Answer from the drawing. Dimensions are ordinates in mm from the lowest x, y and z of the part. A direction names the side the tool comes from. Give positions to 0.01 mm unless a question says otherwise; leave off trailing zeros. Write each loop counter-clockwise with the first axis right and the second up, starting at its lowest first coordinate (ties: lowest second). Pieces come first, ordered by that corner, then holes. Notation, with made-up numbers: (26, 84) -> (49, 84) arc R20 ccw to (49, 88) -> close; hole circle Ø1 at (-20.5, -10). An arc over 180 degrees is marked (long way). Write item = value, one per line.
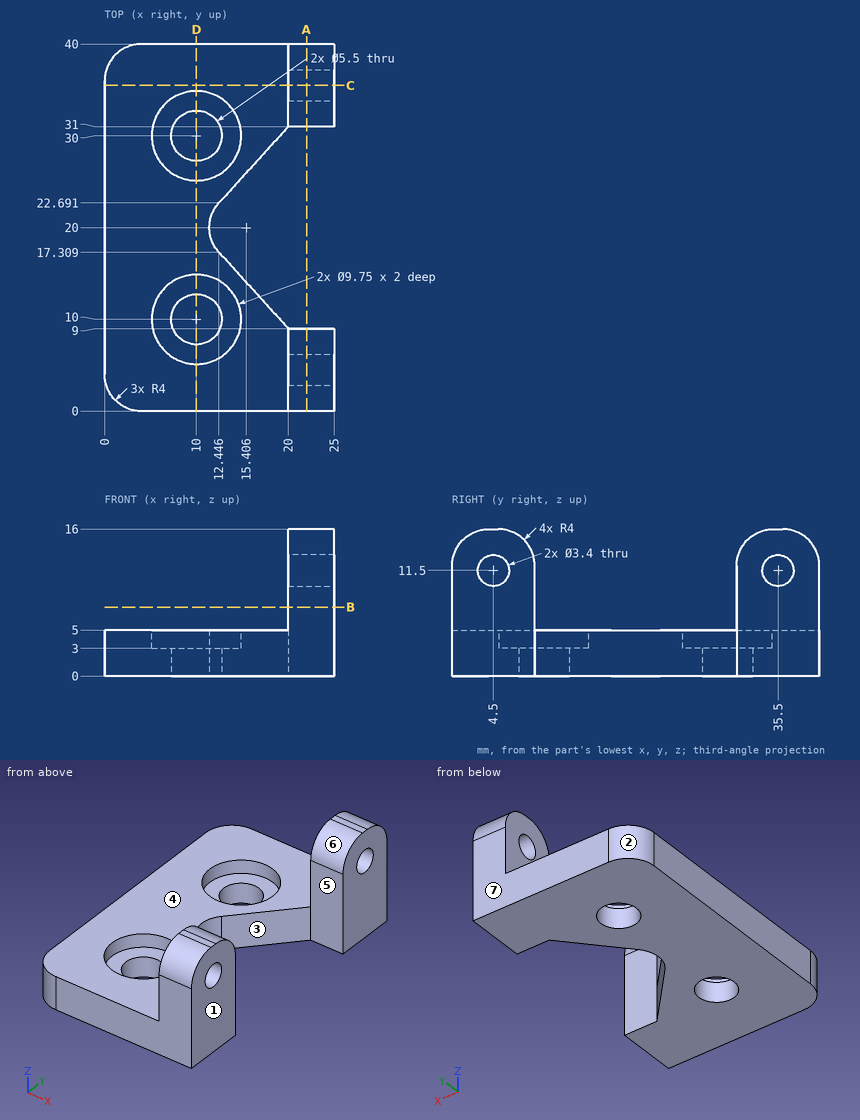
(1) The part is cut by section D-D on x = 10. Count the separate pieces of the cut face and the enclosed holes in it, plus the area to 3 significant figures.
Checks:
separate_pieces = 3
enclosed_holes = 0
area = 128 mm²
(2) A tool of negligible diameter and unlimited length cuts with its end or side. For the marked faces 4, 5, 6 and 7, from which of +Z, -Z, +X, -X, +Y, -Y can it reach the whole face along a straight path? Write none if from no direction.
Checks:
face_4 = +Z, -X, +Y, -Y
face_5 = +Z, -Z, +X
face_6 = +Z, +X, -X
face_7 = +Z, -Z, +X, -X, +Y
(3) Consider L1, parallel to Y at x = 23.7, z = 11.5; L2, parallel to Y at x = 22, z = 1; L3, parallel to Y at x = 12, z = 1.5 (1 decimal). Determine where each line is inside the solid, lowest interval first.
Checks:
L1 = 0 to 2.8, 6.2 to 9, 31 to 33.8, 37.2 to 40
L2 = 0 to 9, 31 to 40
L3 = 0 to 8.1, 11.9 to 17.9, 22.1 to 28.1, 31.9 to 40
(4) The part is cut by section A-A on x = 22. Determine the outline of the cut face in (y, z), plus the area to 3 significant figures.
Checks:
outline = (0, 0) -> (9, 0) -> (9, 12) arc R4 ccw to (5, 16) -> (4, 16) arc R4 ccw to (0, 12) -> close; (31, 0) -> (40, 0) -> (40, 12) arc R4 ccw to (36, 16) -> (35, 16) arc R4 ccw to (31, 12) -> close; hole circle Ø3.4 at (4.5, 11.5); hole circle Ø3.4 at (35.5, 11.5)
area = 256 mm²
(5) For a pull along Y with two mould halves and no side action, classify the marked faces 1, 2 and 3 as released by +Y, released by -Y, zero draft, split by the parting line, or undercut.
Checks:
face_1 = zero draft
face_2 = released by +Y
face_3 = undercut
(6) Given P1, Ø8, axis at x = 10, y = 10, coming from the +Z side; P2, Ø2.5, axis at y = 34.5, z = 13, coming from the -X side; P3, Ø10.5, axis at x = 10, y = 32, coming from the +Z side, each flat-ended and moving along its own axis, determine where each tip first touches the part or whether it passes through.
Checks:
P1 = 3
P2 = 20
P3 = 5
(7) The part is cut by section B-B on z = 7.5. Determine the outline of the cut face in (x, y), plus the area to 3 significant figures.
Checks:
outline = (20, 0) -> (25, 0) -> (25, 9) -> (20, 9) -> close; (20, 31) -> (25, 31) -> (25, 40) -> (20, 40) -> close
area = 90.0 mm²
(8) The part is cut by section C-C on y = 35.5. Determine the outline of the cut face in (x, z).
Checks:
outline = (0, 0) -> (25, 0) -> (25, 9.8) -> (20, 9.8) -> (20, 5) -> (0, 5) -> close; (20, 13.2) -> (25, 13.2) -> (25, 16) -> (20, 16) -> close
